Could you check a few things on this drawing? It's one solid part, dimensions in mm from its lowest x, y, z. A direction names the side the tool comes from. Round coordinates to 2 decimals unless told otherwise and drop trailing zeros. Write each loop counter-clockwise with the first axis right and the second up, starting at its lowest first coordinate (ties: lowest second). Pieces come first, ordered by that corner, then holes. Notation, with made-up numbers: (75, -24) -> (87, -24) arc R8 cw to (87, -19) -> close; hole circle Ø5 at (-18, -13.5). An arc over 180 degrees is marked (long way). Answer in a Markdown table with one row per item.
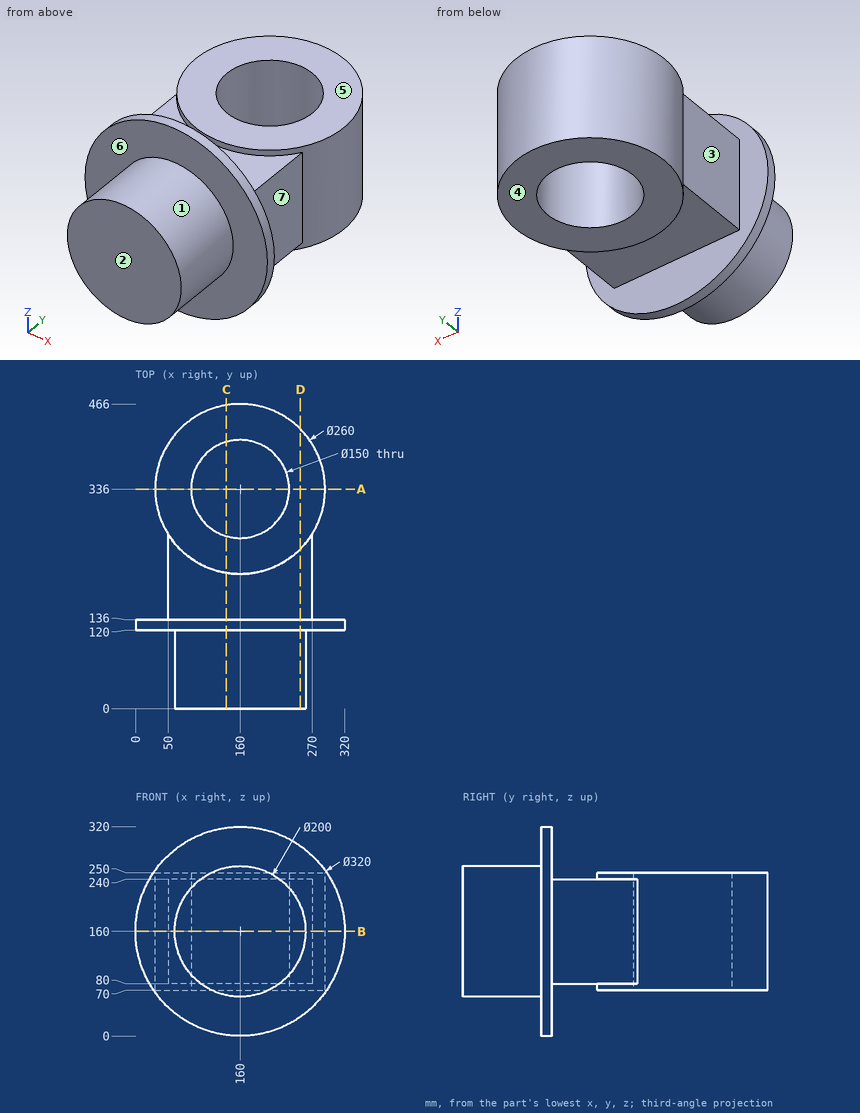
1) I want a section at A-A, the plane y = 336. List the corners of the cut face in (x, z) for me.
Response:
| item | result |
|---|---|
| outline | (30, 70) -> (85, 70) -> (85, 250) -> (30, 250) -> close; (235, 70) -> (290, 70) -> (290, 250) -> (235, 250) -> close |
2) I want a section at D-D, the plane x = 252. List the corners of the cut face in (y, z) for me.
Response:
| item | result |
|---|---|
| outline | (0, 120.81) -> (120, 120.81) -> (120, 29.1) -> (136, 29.1) -> (136, 80) -> (244.15, 80) -> (244.15, 70) -> (427.85, 70) -> (427.85, 250) -> (244.15, 250) -> (244.15, 240) -> (136, 240) -> (136, 290.9) -> (120, 290.9) -> (120, 199.19) -> (0, 199.19) -> close |
3) For pin 1 (1 mm diameter, centred on x = 197, z = 236, fed in from -Y); pin 2 (12 mm diameter, centred on y = 124.5, z = 97, fed in from +X); pin 3 (3 mm diameter, centred on y = 288.5, z = 225, fed in from +X); pin 4 (5 mm diameter, centred on x = 98.5, z = 41.5, fed in from -Y), each with a flat end and sliding along its axis, tell me the tip position at first contact or that it passes through.
Response:
| item | result |
|---|---|
| pin 1 | stops at y = 0 |
| pin 2 | stops at x = 309.5 |
| pin 3 | stops at x = 281.59 |
| pin 4 | stops at y = 120 |
4) I want a section at B-B, the plane z = 160. List the corners of the cut face in (x, y) for me, and give its area (3 significant figures).
Response:
| item | result |
|---|---|
| outline | (0, 120) -> (60, 120) -> (60, 0) -> (260, 0) -> (260, 120) -> (320, 120) -> (320, 136) -> (270, 136) -> (270, 266.72) arc R130 ccw (long way) to (50, 266.72) -> (50, 136) -> (0, 136) -> close; hole circle Ø150 at (160, 336) |
| area | 83,900 mm^2 |
5) I want a section at C-C, the plane x = 139. List the corners of the cut face in (y, z) for me.
Response:
| item | result |
|---|---|
| outline | (0, 62.23) -> (120, 62.23) -> (120, 1.38) -> (136, 1.38) -> (136, 80) -> (207.71, 80) -> (207.71, 70) -> (264, 70) -> (264, 250) -> (207.71, 250) -> (207.71, 240) -> (136, 240) -> (136, 318.62) -> (120, 318.62) -> (120, 257.77) -> (0, 257.77) -> close; (408, 70) -> (464.29, 70) -> (464.29, 250) -> (408, 250) -> close |
6) Which directions (+Z, -Z, +X, -X, +Y, -Y) give clear straight access to the entire face, cutting with the end or side of a thin tool? Please do the marked faces 1, 2, 3 and 4.
Response:
| item | result |
|---|---|
| face 1 | -Y |
| face 2 | +Z, -Z, +X, -X, -Y |
| face 3 | +Z, -Z, -X |
| face 4 | -Z, +X, -X, +Y |
7) I need wall thicknesses on line 1 (X direction, y = 336, z = 167.5); line 2 (Y direction, x = 160, z = 112.5); line 3 (Y direction, x = 124.5, z = 241). Which ranges of each line are inside material? Lowest first, please. Write a range as [from, to].
Response:
| item | result |
|---|---|
| line 1 | x = [30, 85], [235, 290] |
| line 2 | y = [0, 261], [411, 466] |
| line 3 | y = [0, 136], [210.94, 269.93], [402.07, 461.06] |
8) We'd pull the mould along Y, two halves only. Please class the marked faces 5, 6 and 7: +Y half, -Y half, draft (parallel to the pull), parting line (faces both ways), or undercut.
Response:
| item | result |
|---|---|
| face 5 | draft |
| face 6 | -Y half |
| face 7 | undercut |
